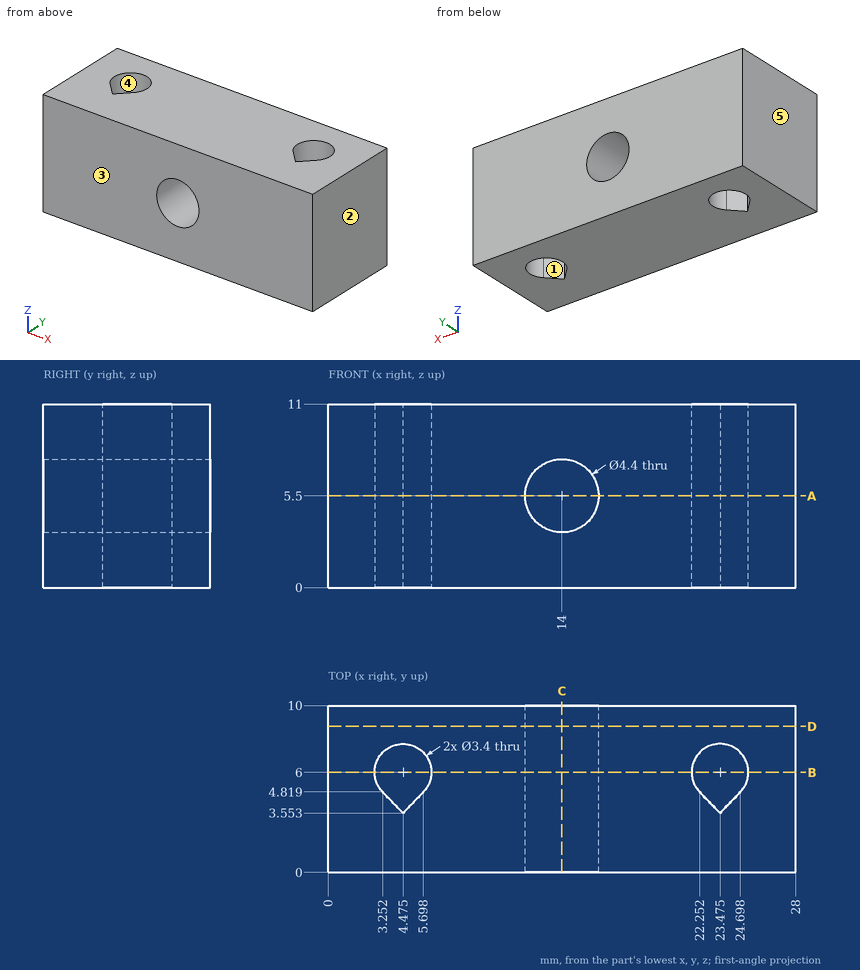
Answer from the drawing. Dimensions are ordinates in mm from the lowest x, y and z of the part. A direction names the side the tool comes from. Give positions to 0.01 mm unless a question says otherwise; leave off trailing zeros. Order: outer loops, then holes, each group sorted by start corner. A loop starts at its lowest first (then second) coordinate and runs counter-clockwise, first axis right, second up.
(1) Find section C-C (x = 14). Give the vertices of the cut face in (y, z), plus the area to 3 significant figures.
(2) Find section A-A (z = 5.5). Give the vertices of the cut face in (x, y) (1 decimal).
(3) Given pin 1 (3 mm diameter, centred on x = 23.475, y = 6, fed in from -Z), flat-ended and moving along its own axis, determine where the tip first touches the part or whether it passes through.
(4) For a pull along Y with two mould halves and no side action, classify the marked faces 3, 4 and 5 as released by +Y, released by -Y, zero draft, split by the parting line, or undercut.
(5) Find section D-D (y = 8.75). Give the vertices of the cut face in (x, z), plus the area to 3 significant figures.
(6) Straight lines are drawn through the part: L1, parallel to Z at x = 14, y = 5.5; L2, parallel to X at y = 6, z = 6.5 (1 decimal); L3, parallel to X at y = 5.5, z = 4.75. For each, find the intervals that lie inside material, in ascending order.
(7) For the marked faces 1 and 2, determine the directions among +Z, -Z, +X, -X, +Y, -Y from which every point of the face is accessible in a straight line to the end or side of a thin tool.
(8) Find section B-B (y = 6). Give the vertices of the cut face in (x, z) (1 decimal).
Result sheet:
1. outline: (0, 0) - (10, 0) - (10, 3.3) - (0, 3.3) - close; (0, 7.7) - (10, 7.7) - (10, 11) - (0, 11) - close
1. area: 66.0 mm2
2. outline: (0, 0) - (11.8, 0) - (11.8, 10) - (0, 10) - close; (16.2, 0) - (28, 0) - (28, 10) - (16.2, 10) - close; hole (3.3, 4.8) - (4.5, 3.6) - (5.7, 4.8) arc R1.7 ccw (long way) to start; hole (22.3, 4.8) - (23.5, 3.6) - (24.7, 4.8) arc R1.7 ccw (long way) to start
3. pin 1: passes through
4. face 3: released by -Y
4. face 4: undercut
4. face 5: zero draft
5. outline: (0, 0) - (28, 0) - (28, 11) - (0, 11) - close; hole circle Ø4.4 at (14, 5.5)
5. area: 293 mm2
6. L1: z = 0 to 3.3, 7.7 to 11
6. L2: x = 0 to 2.8, 6.2 to 12, 16 to 21.8, 25.2 to 28
6. L3: x = 0 to 2.85, 6.1 to 11.93, 16.07 to 21.85, 25.1 to 28
7. face 1: +Z, -Z
7. face 2: +Z, -Z, +X, +Y, -Y
8. outline: (0, 0) - (2.8, 0) - (2.8, 11) - (0, 11) - close; (6.2, 0) - (21.8, 0) - (21.8, 11) - (6.2, 11) - close; (25.2, 0) - (28, 0) - (28, 11) - (25.2, 11) - close; hole circle Ø4.4 at (14, 5.5)
